Source: CAD feature listing. Evaluate the final solid. Frame: model axes, mm. A direction names the side the tool comes from. Coordinates: 2 decimals unless noted, no trailing zeros. Loops run counter-clockwise (first coordinate to the right, second up) from the corner with the lowest first, then second, coordinate; pieces in that order, holes last.
```python
from build123d import *

# Parameters (mm, degrees)
IZIM1_W                     = 19
IZIM1_H                     = 2.55
IZIM4_R                     = 2.575
Y_KSEKLIK_EKSTR_ZYON1_DEPTH = 0.6
IZIM5_R                     = 3.175
Y_KSEKLIK_EKSTR_ZYON2_DEPTH = 1.9
IZIM7_R                     = 2.575
Y_KSEKLIK_EKSTR_ZYON4_DEPTH = 0.6
Y_KSEKLIK_EKSTR_ZYON5_START = 1.9
IZIM8_R                     = 3.175
Y_KSEKLIK_EKSTR_ZYON5_DEPTH = 1.9
IZIM9_R                     = 1.5
KES_EKSTR_ZYON1_DEPTH       = 100
PAH1_SIZE                   = 0.1


# Read off the part's stored shape, not the designer's step: Draft2, Draft3
with BuildPart() as part:
    # Çizim1 → Döndür3 (revolve)
    with BuildSketch(Plane(origin=(0, 0, 0), x_dir=(0, 0, -1), z_dir=(1, 0, 0)), mode=Mode.PRIVATE) as d_nd_r3_sk:
        with Locations((0, -1.275)):
            Rectangle(IZIM1_W, IZIM1_H)
    revolve(d_nd_r3_sk.sketch.rotate(Axis((0, 0, 15.544933078), (0, 0, -1)), 270), axis=Axis((0, 0, 15.544933078), (0, 0, -1)))

    # Çizim4 → Yükseklik-Ekstrüzyon1 (add)
    with BuildSketch(Plane(origin=(0, 0, -9.5), x_dir=(-1, 0, 0), z_dir=(0, 0, -1))):
        Circle(IZIM4_R)
    extrude(amount=Y_KSEKLIK_EKSTR_ZYON1_DEPTH)

    # Çizim5 → Yükseklik-Ekstrüzyon2 (add)
    with BuildSketch(Plane(origin=(0, 0, -10.1), x_dir=(-1, 0, 0), z_dir=(0, 0, -1))):
        with Locations(Location((0, 0, 0), (0, 0, 180))):
            Circle(IZIM5_R)
    extrude(amount=Y_KSEKLIK_EKSTR_ZYON2_DEPTH)

    # Draft2 outline → Draft2 (revolve)
    with BuildSketch(Plane.XZ):
        Polygon((3.175, -10.003459779), (2.575, -9.5), (2.575, -10.1), (3.175, -10.1), align=None)
    revolve(axis=Axis((0, 0, 0), (0, 0, 1)))

    # Çizim7 → Yükseklik-Ekstrüzyon4 (add)
    with BuildSketch(Plane.XY.offset(9.5)):
        Circle(IZIM7_R)
    extrude(amount=Y_KSEKLIK_EKSTR_ZYON4_DEPTH)

    # Çizim8 → Yükseklik-Ekstrüzyon5 (add)
    with BuildSketch(Plane.XY.offset(10.1).offset(Y_KSEKLIK_EKSTR_ZYON5_START)):
        Circle(IZIM8_R)
    extrude(amount=-Y_KSEKLIK_EKSTR_ZYON5_DEPTH)

    # Draft3 outline → Draft3 (revolve)
    with BuildSketch(Plane.XZ):
        Polygon((2.575, 9.5), (3.175, 10.003459779), (3.175, 10.1), (2.575, 10.1), align=None)
    revolve(axis=Axis((0, 0, 0), (0, 0, 1)))

    # Çizim9 → Kes-Ekstrüzyon1 (cut)
    with BuildSketch(Plane.XY.offset(12)):
        Circle(IZIM9_R)
    extrude(amount=-KES_EKSTR_ZYON1_DEPTH, mode=Mode.SUBTRACT)

    # Pah1
    pah1_edges = [part.edges().sort_by_distance(p)[0] for p in [
        (-3.175, 0, -12),
        (-3.175, 0, 12),
    ]]
    chamfer(pah1_edges, length=PAH1_SIZE)


solid = part.part
```
Q1. Material intervals for line 1 along Y through (x, z) = (0, 3.5); line 2 along X through (y, z) = (0.5, 4.75); line 3 along Y through (x, z) = (1, -7.5), sorted ascending.
Q2. First-contact query: pin 1 Ø2 at (y, z) = (0.5, -2.5) entering from -X; pin 2 Ø2 at (x, z) = (-1, 1.5) entering from -Y; pin 3 Ø1 at (y, z) = (0.5, -3) entering from +X. Flat tips, straight axial feed; report the tip coordinate or a pass-through.
Q3. Draft query along X for faces 1 (the cylindrical face through (-0.69, -3.1, 10.97)), 2 (the cylindrical face through (-1.5, 0.07, 0.17)). Return one class per face: released by +X, released by -X, zero draft, split by the parting line, or undercut.
Q4. Reachability of faces 3 (the cylindrical face through (-0.69, -3.1, -10.94)), 4 (the cylindrical face through (2.43, -0.77, -0.13)) from +Z, -Z, +X, -X, +Y, -Y: full face, straight path, thin tool, end or side. Return the list, or none.
Q5. Section query A-A on y = 0. Return the cut outline in (x, z) (3 decimals), then the cut area to 3 significant figures.
Q6. Section query C-C on z = 5.25. Return the cut outline in (x, y), then the cut area to 3 significant figures.
Resolved:
1. line 1: y = -2.55 to -1.5, 1.5 to 2.55
1. line 2: x = -2.5 to -1.41, 1.41 to 2.5
1. line 3: y = -2.35 to -1.12, 1.12 to 2.35
2. pin 1: stops at x = -2.55
2. pin 2: stops at y = -2.55
2. pin 3: stops at x = 2.55
3. face 1: split by the parting line
3. face 2: undercut
4. face 3: +Z, -Z
4. face 4: none
5. outline: (-3.175, -11.9) - (-3.075, -12) - (-1.5, -12) - (-1.5, 12) - (-3.075, 12) - (-3.175, 11.9) - (-3.175, 10.003) - (-2.575, 9.5) - (-2.55, 9.5) - (-2.55, -9.5) - (-2.575, -9.5) - (-3.175, -10.003) - close; (1.5, -12) - (3.075, -12) - (3.175, -11.9) - (3.175, -10.003) - (2.575, -9.5) - (2.55, -9.5) - (2.55, 9.5) - (2.575, 9.5) - (3.175, 10.003) - (3.175, 11.9) - (3.075, 12) - (1.5, 12) - close
5. area: 56.0 mm2
6. outline: circle Ø5.1 at (0, 0); hole circle Ø3 at (0, 0)
6. area: 13.4 mm2
